```python
from build123d import *

# Parameters (mm, degrees)
F0_W     = 50.0062517822
F0_H     = 82.9441100359
F1_DEPTH = 25.4
F2_R     = 5.08
F3_T     = -2.54


# Not quite as in the source:
# - the program builds the solid bodies; features that only make, move or delete a surface that nothing else refers to are left out


with BuildPart() as f1:
    # F0 (on Front) → F1 (new body)
    with BuildSketch(Plane.XZ):
        with Locations((47.5059393793, 78.971914947)):
            Rectangle(F0_W, F0_H)
    extrude(amount=F1_DEPTH)

    # F2
    f2_edges = [f1.edges().sort_by_distance(p)[0] for p in [
        (72.509065, -25.4, 78.971915),
        (22.502813, -25.4, 78.971915),
        (47.505939, -25.4, 120.44397),
        (47.505939, -25.4, 37.49986),
    ]]
    fillet(f2_edges, radius=F2_R)

    # F3
    f3_openings = [f1.faces().sort_by_distance(p)[0] for p in [
        (47.505939, 0, 78.971915),
    ]]
    offset(amount=F3_T, openings=f3_openings)


solid = f1.part
```
Can you work these out from the model? Positions are in its coordinate system, mm. A direction names the side the tool comes from. Coordinates: 2 decimals unless noted, no trailing zeros. Loops run counter-clockwise (first coordinate to the right, second up) from the corner with the lowest first, then second, coordinate; pieces in that order, holes last. Notation, with made-up numbers: (35.25, 51.25) -> (88.25, 51.25) arc R27 cw to (88.25, 81.25) -> close; hole circle Ø8 at (27, 22.25). An arc over 180 degrees is marked (long way). Put each result on its own line as item: value. Start each with the question number.
Q1. If I drill on line 1 (Z direction, x = 40, y = -5.25); line 2 (X direction, y = -13.25, z = 71); line 3 (Y direction, x = 29, z = 90), over which ranges is the centre line in solid material (lowest first)? Write a range as [from, to].
Q2. I want a section at A-A (y = -12). Write out the boundary of the cut face in (x, z).
Q3. Thinking about a two-plate mould opening in X: for faces 1 (the face through (69.24, -22.1, 79.52)), 2 (the face through (23, 0, 79)), 3 (the face through (72.509, -10, 78)), 4 (the face through (23.95, -23.87, 79.55)), which applies, pulls with the +X half, pulls with the -X half, needs draft (parallel to the pull), parting line crosses it, or undercut?
Q4. For faces 5 (the face through (47, -10, 120.444)), 6 (the face through (47, -10, 117.904)), which set-ups out of +Z, -Z, +X, -X, +Y, -Y let a thin tool reach every point of the face, with its end or its side?
Q5. I want a section at B-B (x = 42). Write out the boundary of the cut face in (y, z).
Q6. I'm going to push a flat-ended pin straight in: P1, Ø2, axis at x = 52.5, z = 67, coming from the +Y side. Where does the tip first touch, or does it pass through?
Q7. I want a section at C-C (z = 51). Write out the boundary of the cut face in (x, y), plus the area to 3 significant figures.
Taken from the geometry:
1. line 1: z = [37.5, 40.04], [117.9, 120.44]
1. line 2: x = [22.5, 25.04], [69.97, 72.51]
1. line 3: y = [-25.4, -22.86]
2. outline: (22.5, 37.5) -> (72.51, 37.5) -> (72.51, 120.44) -> (22.5, 120.44) -> close; hole (25.04, 40.04) -> (69.97, 40.04) -> (69.97, 117.9) -> (25.04, 117.9) -> close
3. face 1: undercut
3. face 2: needs draft
3. face 3: pulls with the +X half
3. face 4: pulls with the -X half
4. face 5: +Z, +X, -X, +Y, -Y
4. face 6: +Y
5. outline: (-25.4, 42.58) arc R5.08 ccw to (-20.32, 37.5) -> (0, 37.5) -> (0, 40.04) -> (-20.32, 40.04) arc R2.54 cw to (-22.86, 42.58) -> (-22.86, 115.36) arc R2.54 cw to (-20.32, 117.9) -> (0, 117.9) -> (0, 120.44) -> (-20.32, 120.44) arc R5.08 ccw to (-25.4, 115.36) -> close
6. P1: stops at y = -22.86
7. outline: (22.5, -20.32) arc R5.08 ccw to (27.58, -25.4) -> (67.43, -25.4) arc R5.08 ccw to (72.51, -20.32) -> (72.51, 0) -> (69.97, 0) -> (69.97, -20.32) arc R2.54 cw to (67.43, -22.86) -> (27.58, -22.86) arc R2.54 cw to (25.04, -20.32) -> (25.04, 0) -> (22.5, 0) -> close
7. area: 235 mm2
